Verification items for the finished model (mm, model axes). A direction names the side the tool comes from. Round coordinates to 2 decimals unless told otherwise and drop trailing zeros. Loops run counter-clockwise (first coordinate to the right, second up) from the corner with the lowest first, then second, coordinate; pieces in that order, holes last. Notation, with made-up numbers: M -20.75,-19.75 L 36.25,-19.75 A32 ccw 36.25,12.25 Z; hole C 9,50.5 d5. An arc over 180 degrees is marked long. Write item = value, one per line. Start each with the question number.
from build123d import *

# Parameters (mm, degrees)
F2_R        = 1
F3_DEPTH    = 10
F4_R        = 3.5
F4_R_2      = 2
F5_DEPTH    = 1
F6_DEPTH    = 35
F7_S5_R     = 2
F7_T6_DEPTH = 6
F8_R        = 0.49999
F9_R        = 7
F10_SIZE    = 1
F11_R       = 1
F12_DEPTH   = 35


# Not quite as in the source:
# - a fillet or chamfer that OpenCascade refuses, or shapes differently, is made with other operations: its cross-section is extruded or revolved along the edge and cut away or added
# - a fillet or chamfer is up to 0.001 mm smaller than in the source, because OpenCascade refuses the exact size


with BuildPart() as f1:
    # F0 (on Front) → F1 (revolve)
    with BuildSketch(Plane.XZ):
        Polygon((-6, 0), (0, 0), (0, 40.6942627281), (-3, 40.6942627281), (-3, 28.6942627281), (-6, 25.2438845978), (-9.1123259154, 12.6219422989), align=None)
    revolve(axis=Axis((0, 0, 20.347131364), (0, 0, -1)))

    # F2 (on Top) → F3 (cut)
    with BuildSketch(Plane.XY):
        Circle(F2_R)
    extrude(amount=F3_DEPTH, mode=Mode.SUBTRACT)

    # F4 (on face) → F5 (join)
    with BuildSketch(Plane.XY.offset(40.6942627281)):
        Circle(F4_R)
        Circle(F4_R_2, mode=Mode.SUBTRACT)
    extrude(amount=F5_DEPTH)

    # F6 (cut): a face of the model
    f6_faces = [f1.faces().sort_by_distance(p)[0] for p in [
        (0, 0, 40.6942627281),
    ]]
    extrude(f6_faces, amount=-F6_DEPTH, mode=Mode.SUBTRACT)

    # F7: chamfer of 2 on 1 edges, made by hand


with BuildPart() as f7_tool2:
    # F7_s3 → F7_t4 (revolve)
    with BuildSketch(Plane.XZ):
        Polygon((1, 3.6942627281), (3, 5.6942627281), (1, 5.6942627281), align=None)
    revolve(axis=Axis((0, 0, 5.6942627281), (0, 0, -1)))

    # F7_s5 → F7_t6 (intersect, symmetric)
    with BuildSketch(Plane.XY.offset(4.7)):
        Circle(F7_S5_R)
    extrude(amount=F7_T6_DEPTH, both=True, mode=Mode.INTERSECT)


with BuildPart() as f1_1:
    add(f1.part)

    # F7_t1: cut F7_tool2
    add(f7_tool2.part, mode=Mode.SUBTRACT)

    # F8 (radius 0.5 in the source; OpenCascade refuses exactly that, so slightly less here)
    f8_edges = [f1_1.edges().sort_by_distance(p)[0] for p in [
        (-3.5, 0, 41.694263),
        (-3.5, 0, 40.694263),
    ]]
    fillet(f8_edges, radius=F8_R)

    # F9
    f9_edges = [f1_1.edges().sort_by_distance(p)[0] for p in [
        (3, 0, 28.694263),
        (6, 0, 25.243885),
        (9.112326, 0, 12.621942),
    ]]
    fillet(f9_edges, radius=F9_R)

    # F10
    f10_edges = [f1_1.edges().sort_by_distance(p)[0] for p in [
        (6, 0, 0),
    ]]
    chamfer(f10_edges, length=F10_SIZE)

    # F11 (on face) → F12 (cut)
    with BuildSketch(Plane.XY.offset(41.6942627281)):
        with Locations((-6.5546142869, 0)):
            Circle(F11_R)
    extrude(amount=-F12_DEPTH, mode=Mode.SUBTRACT)


solid = f1_1.part
1. Tool access check on faces 5 (the flat face through (0.1, 1.2, 0)), 6 (the cylindrical face through (-2.77, -1.15, 35.94)). Record the directions out of +Z, -Z, +X, -X, +Y, -Y that give a thin tool (end or side, any length) a straight path to the whole face; none if there is none.
2. Gauge pin test, flat ends, axial feed: P1, Ø0.6, axis at x = -6.5, y = 0, coming from the +Z side; P2, Ø2.5, axis at x = -6.55, y = 0, coming from the +Z side; P3, Ø2, axis at y = -5.5, z = 19, coming from the -X side; P4, Ø2, axis at y = 5, z = 30, coming from the +X side. Record the tip position at first contact, or that the pin passes through.
3. Mould release check, pull along Y, two halves, no side actions. Record for faces 1 (the cylindrical face through (0, -2, 23)), 2 (the flat face through (1, -2, 41.694)), 3 (the cylindrical face through (-5.6, 0.3, 14.2)), 4 (the conical face through (-6.38, -2.64, 3.67)): pulls with the +Y half, pulls with the -Y half, needs draft (parallel to the pull), parting line crosses it, or undercut.
4. Section check A-A, the plane z = 35. Enter the section's corners in (x, y), and give its area (3 significant figures).
5. Thickness scan on line 1 (X direction, y = -7.25, z = 14.5); line 2 (X direction, y = 0, z = 2.95); line 3 (Y direction, x = 0.75, z = 13). Record the ranges inside material, lowest first.
Computed values:
q1.face_5 = -Z, +X, -X, +Y, -Y
q1.face_6 = none
q2.P1 = 6.69
q2.P2 = 26
q2.P3 = -6.11
q2.P4 = through
q3.face_1 = undercut
q3.face_2 = needs draft
q3.face_3 = undercut
q3.face_4 = parting line crosses it
q4.outline = C 0,0 d6; hole C 0,0 d4
q4.area = 15.7 mm2
q5.line_1 = -4.72 to 4.72
q5.line_2 = -6.73 to -1, 1 to 6.73
q5.line_3 = -8.86 to -1.85, 1.85 to 8.86
